Input: part model. Units: mm. Frame: model coordinates. A direction names the side the tool comes from. Coordinates: 2 decimals unless noted, no trailing zeros. Order: outer loops, then holes, each group sorted by start corner. A loop starts at its lowest first (then second) coordinate and runs counter-clockwise, first axis right, second up. Notation, with made-up numbers: M 22,-4 L 28,-4 A12 cw 28,12 Z; hole C 69,66 d8. An arc over 180 degrees is marked long. Answer in a Markdown table with one row per item.
from build123d import *

# Parameters (mm, degrees)
SKETCH2_R           = 3.81
BOSS_EXTRUDE1_DEPTH = 12.7
BOSS_EXTRUDE2_DEPTH = 127
SKETCH4_R           = 3.556
BOSS_EXTRUDE3_DEPTH = 5.08
FILLET3_R           = 0.254
SKETCH5_R           = 1.27
CUT_EXTRUDE1_DEPTH  = 0.254


with BuildPart() as part:
    # Sketch2 → Boss-Extrude1 (new body)
    with BuildSketch(Plane(origin=(0, 0, 0), x_dir=(1, 0, 0), z_dir=(0, 1, 0))):
        with Locations(Location((0, 0, 0), (0, 0, 270))):
            Circle(SKETCH2_R)
    extrude(amount=BOSS_EXTRUDE1_DEPTH)

    # Sketch3 → Boss-Extrude2 (add)
    with BuildSketch(Plane(origin=(0, 12.7, 0), x_dir=(1, 0, 0), z_dir=(0, 1, 0))):
        Polygon((3.81, 0), (3.082354749, 2.239461811), (1.177354749, 3.623525327), (-1.177354749, 3.623525327), (-3.082354749, 2.239461811), (-3.81, 0), (-3.082354749, -2.239461811), (-1.177354749, -3.623525327), (1.177354749, -3.623525327), (3.082354749, -2.239461811), align=None)
    extrude(amount=BOSS_EXTRUDE2_DEPTH)

    # Sketch4 → Boss-Extrude3 (add)
    with BuildSketch(Plane.XZ):
        with Locations(Location((0, 0, 0), (0, 0, 270))):
            Circle(SKETCH4_R)
    extrude(amount=BOSS_EXTRUDE3_DEPTH)

    # Fillet3
    fillet3_edges = [part.edges().sort_by_distance(p)[0] for p in [
        (0, -5.08, 3.556),
    ]]
    fillet(fillet3_edges, radius=FILLET3_R)

    # Sketch5 → Cut-Extrude1 (cut)
    with BuildSketch(Plane(origin=(0, 139.7, 0), x_dir=(1, 0, 0), z_dir=(0, 1, 0))):
        with Locations(Location((0, 0, 0), (0, 0, 270))):
            Circle(SKETCH5_R)
    extrude(amount=-CUT_EXTRUDE1_DEPTH, mode=Mode.SUBTRACT)


solid = part.part
1) Reachability of faces 1 (the face through (-3.47, -2.38, 0.77)), 2 (the face through (3.451, 75.311, -1.104)), 3 (the face through (3.44, 75.31, 1.14)), 4 (the face through (-3.44, 75.31, -1.14)), 5 (the face through (-3.451, 75.311, 1.104)) from +Z, -Z, +X, -X, +Y, -Y: full face, straight path, thin tool, end or side. Return the list, or none.
Resolved:
| item | result |
|---|---|
| face 1 | -Y |
| face 2 | -Z, +X, +Y |
| face 3 | +Z, +X, +Y |
| face 4 | -Z, -X, +Y |
| face 5 | +Z, -X, +Y |
2) Cut plane B-B, the plane y = 43. Output: boundary loops of the cut face in (x, z), and give its area (3 significant figures).
Resolved:
| item | result |
|---|---|
| outline | M -3.81,0 L -3.08,-2.24 L -1.18,-3.62 L 1.18,-3.62 L 3.08,-2.24 L 3.81,0 L 3.08,2.24 L 1.18,3.62 L -1.18,3.62 L -3.08,2.24 Z |
| area | 42.7 mm2 |
3) Mould query, pull axis Z, two halves, no side actions, for faces 6 (the face through (3.778, 6.261, -0.496)), 7 (the face through (0, 75, 3.624)), 8 (the face through (0, 139.446, 0)). Classes: +Z half, -Z half, draft (parallel to the pull), parting line (faces both ways), or undercut.
Resolved:
| item | result |
|---|---|
| face 6 | parting line |
| face 7 | +Z half |
| face 8 | undercut |
4) Material intervals for probe 1 along X at (y, z) = (139.6, 0); probe 2 along Z at (x, y) = (0.25, 98.5); probe 3 along Y at (x, z) = (-3.25, 1), sorted ascending.
Resolved:
| item | result |
|---|---|
| probe 1 | x = -3.81 to -1.27, 1.27 to 3.81 |
| probe 2 | z = -3.62 to 3.62 |
| probe 3 | y = -5.06 to 139.7 |
5) Cut plane A-A, the plane x = 0. Output: boundary loops of the cut face in (y, z).
Resolved:
| item | result |
|---|---|
| outline | M -5.08,-3.3 A0.25 ccw -4.83,-3.56 L 0,-3.56 L 0,-3.81 L 12.7,-3.81 L 12.7,-3.62 L 139.7,-3.62 L 139.7,-1.27 L 139.45,-1.27 L 139.45,1.27 L 139.7,1.27 L 139.7,3.62 L 12.7,3.62 L 12.7,3.81 L 0,3.81 L 0,3.56 L -4.83,3.56 A0.25 ccw -5.08,3.3 Z |
6) Contact query for flat-ended pins moving along their axis: pin 1 (2.5 mm diameter, centred on x = 0.5, y = 77, fed in from +Z); pin 2 (1.9 mm diameter, centred on x = 0.5, y = 73, fed in from -Z); pin 3 (2 mm diameter, centred on y = 86.5, z = -2.5, fed in from -X). Output: stop coordinate, or through.
Resolved:
| item | result |
|---|---|
| pin 1 | stops at z = 3.62 |
| pin 2 | stops at z = -3.62 |
| pin 3 | stops at x = -3.32 |
